Here's how the part is built. I have some questions about the finished solid (model axes, mm). A direction names the side the tool comes from. Round coordinates to 2 decimals unless told otherwise and drop trailing zeros. Order: outer loops, then holes, each group sorted by start corner. A loop starts at its lowest first (then second) coordinate and runs counter-clockwise, first axis right, second up. Notation, with made-up numbers: M 11,-40 L 35,-40 A30 cw 35,-11 Z; hole C 44,80.25 d4. An arc over 180 degrees is marked long. Use one line per item in the form item = value. Start each with the question number.
```python
from build123d import *

# Parameters (mm, degrees)
SKETCH1_W             = 50.8
SKETCH1_H             = 76.2
BOSS_EXTRUDE1_DEPTH   = 1000
SKETCH2_W             = 46.8
SKETCH2_H             = 72.2
CUT_EXTRUDE1_DEPTH    = 1002.04783602
FILLET2_R             = 2
CROQUIS2_R            = 2.5
CORTAR_EXTRUIR2_DEPTH = 10
CROQUIS3_R            = 2.5
CORTAR_EXTRUIR3_DEPTH = 10
CROQUIS4_R            = 2.5
CORTAR_EXTRUIR4_DEPTH = 10
CROQUIS5_R            = 2.5
CORTAR_EXTRUIR5_DEPTH = 10
CROQUIS6_R            = 2.5
CORTAR_EXTRUIR6_DEPTH = 1004.220613823
MATRIZL1_COUNT        = 12
MATRIZL1_PITCH        = 60
CROQUIS7_R            = 2.5
CORTAR_EXTRUIR7_DEPTH = 10


with BuildPart() as part:
    # Sketch1 → Boss-Extrude1 (new body)
    with BuildSketch(Plane(origin=(0, 0, 0), x_dir=(0, 0, -1), z_dir=(1, 0, 0))):
        Rectangle(SKETCH1_W, SKETCH1_H)
    extrude(amount=-BOSS_EXTRUDE1_DEPTH)

    # Sketch2 → Cut-Extrude1 (cut, through all)
    with BuildSketch(Plane(origin=(0, 0, 0), x_dir=(0, 0, -1), z_dir=(1, 0, 0))):
        Rectangle(SKETCH2_W, SKETCH2_H)
    extrude(amount=-CUT_EXTRUDE1_DEPTH, mode=Mode.SUBTRACT)

    # Fillet2
    fillet2_edges = [part.edges().sort_by_distance(p)[0] for p in [
        (-500, -36.1, 23.4),
        (-500, 36.1, 23.4),
        (-500, 36.1, -23.4),
        (-500, -36.1, -23.4),
        (-500, 38.1, 25.4),
        (-500, 38.1, -25.4),
        (-500, -38.1, -25.4),
        (-500, -38.1, 25.4),
    ]]
    fillet(fillet2_edges, radius=FILLET2_R)

    # Croquis2 → Cortar-Extruir2 (cut)
    with BuildSketch(Plane.XZ.offset(38.1)):
        with Locations(Location((-61.2, 15.4, 0), (0, 0, 270))):
            Circle(CROQUIS2_R)
        with Locations(Location((-38.1, 0, 0), (0, 0, 270))):
            Circle(CROQUIS2_R)
        with Locations(Location((-61.2, -15.4, 0), (0, 0, 270))):
            Circle(CROQUIS2_R)
        with Locations(Location((-15, -15.4, 0), (0, 0, 270))):
            Circle(CROQUIS2_R)
        with Locations(Location((-15, 15.4, 0), (0, 0, 270))):
            Circle(CROQUIS2_R)
    extrude(amount=-CORTAR_EXTRUIR2_DEPTH, mode=Mode.SUBTRACT)

    # Croquis3 → Cortar-Extruir3 (cut)
    with BuildSketch(Plane.XZ.offset(38.1)):
        with Locations(Location((-985, 15.4, 0), (0, 0, 270))):
            Circle(CROQUIS3_R)
        with Locations(Location((-938.8, 15.4, 0), (0, 0, 270))):
            Circle(CROQUIS3_R)
        with Locations(Location((-961.9, 0, 0), (0, 0, 270))):
            Circle(CROQUIS3_R)
        with Locations(Location((-985, -15.4, 0), (0, 0, 270))):
            Circle(CROQUIS3_R)
        with Locations(Location((-938.8, -15.4, 0), (0, 0, 270))):
            Circle(CROQUIS3_R)
    extrude(amount=-CORTAR_EXTRUIR3_DEPTH, mode=Mode.SUBTRACT)

    # Croquis4 → Cortar-Extruir4 (cut)
    with BuildSketch(Plane(origin=(0, 38.1, 0), x_dir=(1, 0, 0), z_dir=(0, 1, 0))):
        with Locations(Location((-853.5, 16.4, 0), (0, 0, 270))):
            Circle(CROQUIS4_R)
        with Locations(Location((-853.5, -16.4, 0), (0, 0, 270))):
            Circle(CROQUIS4_R)
        with Locations(Location((-871, 0, 0), (0, 0, 270))):
            Circle(CROQUIS4_R)
    extrude(amount=-CORTAR_EXTRUIR4_DEPTH, mode=Mode.SUBTRACT)

    # Croquis5 → Cortar-Extruir5 (cut)
    with BuildSketch(Plane(origin=(0, 38.1, 0), x_dir=(1, 0, 0), z_dir=(0, 1, 0))):
        with Locations(Location((-186, 17.9, 0), (0, 0, 270))):
            Circle(CROQUIS5_R)
        with Locations(Location((-186, -17.9, 0), (0, 0, 270))):
            Circle(CROQUIS5_R)
        with Locations(Location((-123, -17.9, 0), (0, 0, 270))):
            Circle(CROQUIS5_R)
        with Locations(Location((-123, 17.9, 0), (0, 0, 270))):
            Circle(CROQUIS5_R)
        with Locations(Location((-65, 17.9, 0), (0, 0, 270))):
            Circle(CROQUIS5_R)
        with Locations(Location((-65, -17.9, 0), (0, 0, 270))):
            Circle(CROQUIS5_R)
    extrude(amount=-CORTAR_EXTRUIR5_DEPTH, mode=Mode.SUBTRACT)

    # Croquis6 → Cortar-Extruir6 (cut, through all)
    with BuildSketch(Plane(origin=(0, 38.1, 0), x_dir=(1, 0, 0), z_dir=(0, 1, 0))):
        with Locations(Location((-179, 0, 0), (0, 0, 270))):
            Circle(CROQUIS6_R)
    cortar_extruir6 = extrude(amount=-CORTAR_EXTRUIR6_DEPTH, mode=Mode.SUBTRACT)

    # MatrizL1: Cortar-Extruir6 ×12
    with Locations(*[(-i * MATRIZL1_PITCH, 0, 0) for i in range(1, MATRIZL1_COUNT)]):
        add(cortar_extruir6, mode=Mode.SUBTRACT)

    # Croquis7 → Cortar-Extruir7 (cut)
    with BuildSketch(Plane(origin=(0, 0, -25.4), x_dir=(-1, 0, 0), z_dir=(0, 0, -1))):
        with Locations(Location((75, -18.1, 0), (0, 0, 90))):
            Circle(CROQUIS7_R)
        with Locations(Location((355, -18.1, 0), (0, 0, 90))):
            Circle(CROQUIS7_R)
        with Locations(Location((635, -18.1, 0), (0, 0, 90))):
            Circle(CROQUIS7_R)
        with Locations(Location((915, -18.1, 0), (0, 0, 90))):
            Circle(CROQUIS7_R)
        with Locations(Location((265, 8.1, 0), (0, 0, 90))):
            Circle(CROQUIS7_R)
        with Locations(Location((830, 8.1, 0), (0, 0, 90))):
            Circle(CROQUIS7_R)
    extrude(amount=-CORTAR_EXTRUIR7_DEPTH, mode=Mode.SUBTRACT)


solid = part.part
```
1) If we section it at A-A on y = -6.5: Write out the boundary of the cut face in (x, z), then the cut area to 3 significant figures.
2) If I drill on line 1 (X direction, y = 37, z = 17); line 2 (X direction, y = -36.6, z = 15.4); line 3 (Y direction, x = -848, z = 17.5), over which ranges is the centre line in solid material (lowest first)?
3) Will these pins go through, and if not, where does the flat tip stop? pin 1 Ø8 at (y, z) = (-24.5, 16.5) entering from -X; pin 2 Ø4.5 at (x, z) = (-938.8, 15.4) entering from -Y.
4) On a 3-axis mill with a long thin cutter (end or side, diameter ignored), from which of +Z, -Z, +X, -X, +Y, -Y can I reach the whole of each face in a straight line? I mean faces 1 (the flat face through (-493, -36.1, 0)), 2 (the flat face through (-493, -1, -25.4)). Say none if no direction works.
5) If we mould it in two halves opening along Y, with no side actions, what happens to faces 3 (the flat face through (-1000, 0, 25)), 4 (the flat face through (-493, -38.1, 0)), 5 (the flat face through (-493, 0, -23.4))? For each: +Y half, -Y half, draft (parallel to the pull), parting line (faces both ways), or undercut.
6) If we section it at B-B on x = -377: Write out the boundary of the cut face in (y, z), then the cut area to 3 significant figures.
Completed:
q1.outline = M -1000,-25.4 L 0,-25.4 L 0,-23.4 L -1000,-23.4 Z; M -1000,23.4 L 0,23.4 L 0,25.4 L -1000,25.4 Z
q1.area = 4,000 mm²
q2.line_1 = -1000 to -855.93, -851.07 to -188.33, -183.67 to -125.33, -120.67 to -67.33, -62.67 to 0
q2.line_2 = -1000 to -987.5, -982.5 to -941.3, -936.3 to -63.7, -58.7 to -17.5, -12.5 to 0
q2.line_3 = -38.1 to -36.1, 36.1 to 38.1
q3.pin_1 = through
q3.pin_2 = 36.1
q4.face_1 = +X, -X
q4.face_2 = -Z, +X, -X, +Y, -Y
q5.face_3 = draft
q5.face_4 = -Y half
q5.face_5 = undercut
q6.outline = M -38.1,-23.4 A2 ccw -36.1,-25.4 L 36.1,-25.4 A2 ccw 38.1,-23.4 L 38.1,23.4 A2 ccw 36.1,25.4 L -36.1,25.4 A2 ccw -38.1,23.4 Z; hole M -36.1,-21.4 A2 ccw -34.1,-23.4 L 34.1,-23.4 A2 ccw 36.1,-21.4 L 36.1,21.4 A2 ccw 34.1,23.4 L -34.1,23.4 A2 ccw -36.1,21.4 Z
q6.area = 492 mm²
